Source: CAD feature listing. Evaluate the final solid. Frame: model axes, mm. Give positions to 0.01 mm unless a question says otherwise; leave off trailing zeros. Loops run counter-clockwise (first coordinate to the right, second up) from the corner with the lowest first, then second, coordinate; pieces in that order, holes last. Notation, with made-up numbers: (45, 29) -> (73, 29) arc R33 ccw to (73, 57) -> close; hole circle Ø10 at (88.5, 69). An arc over 180 degrees is marked (long way). Put each result on its own line as item: value.
```python
from build123d import *

# Parameters (mm, degrees)
F0_W     = 838.2
F0_H     = 1676.4
F1_DEPTH = 762
F2_W     = 838.2
F2_H     = 12.7
F3_DEPTH = 50.8
F5_R     = 9.525


with BuildPart() as f1:
    # F0 (on Front) → F1 (new body)
    with BuildSketch(Plane.XZ):
        with Locations((419.1, 838.2)):
            Rectangle(F0_W, F0_H)
    extrude(amount=F1_DEPTH)

    # F2 (on face) → F3 (cut)
    with BuildSketch(Plane.XZ.offset(762)):
        with Locations((419.1, 1060.45)):
            Rectangle(F2_W, F2_H)
    extrude(amount=-F3_DEPTH, mode=Mode.SUBTRACT)

    # F7: sweep along a path in F6
    with BuildLine(Plane(origin=(76.2, 0, 0), x_dir=(0, -1, 0), z_dir=(-1, 0, 0))) as f7_path:
        Line((762, 1600.2), (782.7021915694, 1600.2))
        ThreePointArc((782.7021915694, 1600.2), (797.2096140296, 1595.6493331683), (806.5187336391, 1583.6279286268))
        ThreePointArc((806.5187336391, 1583.6279286268), (844.55, 1371.6), (806.5187336391, 1159.5720713732))
        ThreePointArc((806.5187336391, 1159.5720713732), (797.2096140296, 1147.5506668317), (782.7021915694, 1143))
        Line((782.7021915694, 1143), (762, 1143))
    # F5 (on face) → F7 (sweep)
    with BuildSketch(Plane.XZ.offset(762)):
        with Locations((76.2, 1600.2)):
            Circle(F5_R)
    f7 = sweep(path=f7_path.line)

    # F8: F7 across face
    add(f7.mirror(Plane(origin=(419.1, -736.6, 1054.1), x_dir=(1, 0, 0), z_dir=(0, 0, 1))))


solid = f1.part
```
(1) Section B-B on z = 477. Return loops of the section in (x, y), then the cut area to 3 significant figures.
Calculated:
outline: (0, -762) -> (838.2, -762) -> (838.2, 0) -> (0, 0) -> close
area: 639,000 mm²
(2) Draft query along Z for faces 1 (the flat face through (413, 0, 850)), 2 (the flat face through (413, -737, 1054.1)), 3 (the flat face through (413, -737, 1066.8)), 4 (the flat face through (413, -376, 0)). Return one class per face: released by +Z, released by -Z, zero draft, split by the parting line, or undercut.
Calculated:
face 1: zero draft
face 2: undercut
face 3: undercut
face 4: released by -Z
(3) Line query: probe 1 along Z at (x, y) = (654.5, -757); probe 2 along Y at (x, z) = (256.5, 1607). Output: solid intervals per line, ascending. Write a range as from..to.
Calculated:
probe 1: z = 0..1054.1, 1066.8..1676.4
probe 2: y = -762..0
(4) Section A-A on x = 577.5. Return loops of the section in (y, z), then the cut area to 3 significant figures.
Calculated:
outline: (-762, 0) -> (0, 0) -> (0, 1676.4) -> (-762, 1676.4) -> (-762, 1066.8) -> (-711.2, 1066.8) -> (-711.2, 1054.1) -> (-762, 1054.1) -> close
area: 1,280,000 mm²
(5) First-contact query: P1, Ø6, axis at x = 490, z = 1198, coming from the -Y side; P2, Ø6.5, axis at x = 592, z = 1059.5, coming from the -Y side. Flat tips, straight axial feed; report the tip coordinate or a pass-through.
Calculated:
P1: stops at y = -762
P2: stops at y = -711.2
